Study the drawing (mm; zero at the part's minimum x, y, z) and answer. A direction names the side the tool comes from. Coordinates: 2 decimals unless noted, no trailing zeros. Loops run counter-clockwise (first coordinate to the right, second up) from the corner with the lowest first, then second, coordinate; pieces in that order, holes last. Notation, with made-up numbers: (70.25, -14) - (106.25, -14) arc R24 cw to (106.25, 24) - close; hole circle Ø3 at (55, -39.5). An arc over 180 degrees is marked (long way). Use one line per item in the form item = value.
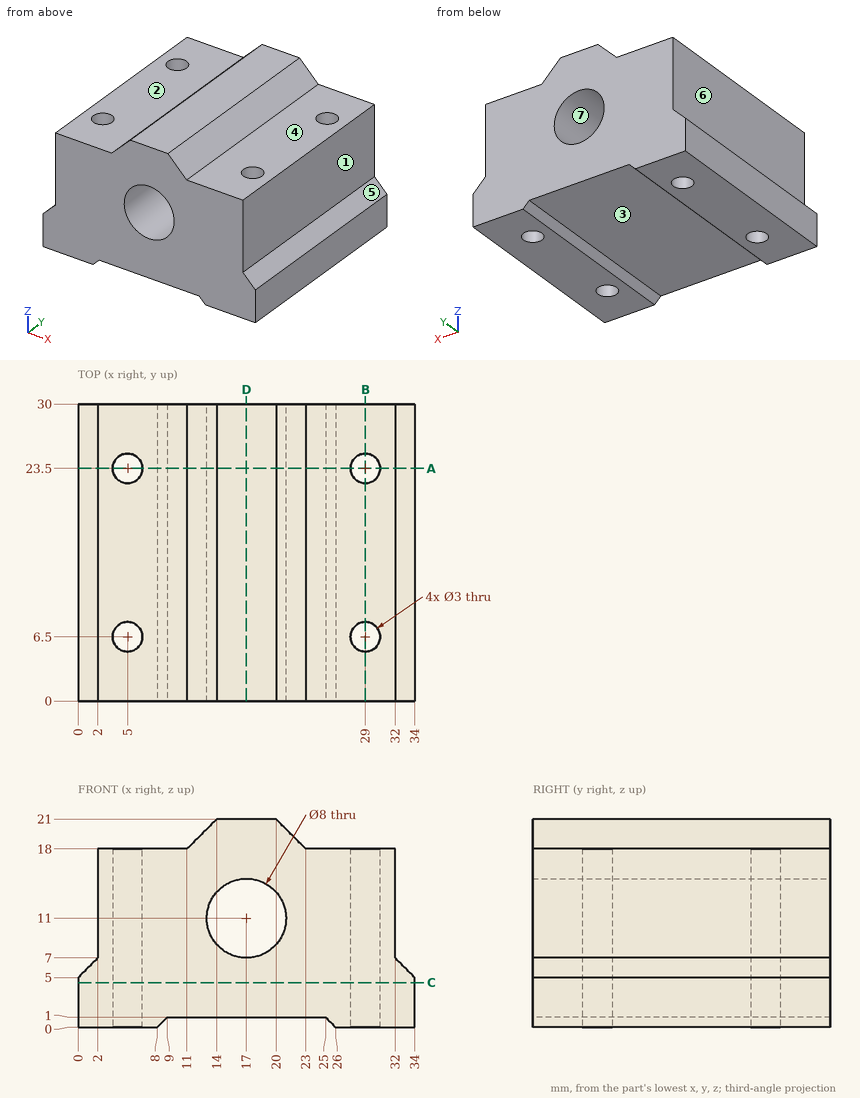
Item 1: Which of the six approach directions +Z, -Z, +X, -X, +Y, -Y give full straight-line access (tool end or side, diameter ignored) to the marked faces 1, 2 and 3?
Results below:
face_1 = +Z, +X, +Y, -Y
face_2 = +Z, -X, +Y, -Y
face_3 = -Z, +Y, -Y
Item 2: Find the intervals of material crossed by L1, parallel to Y at x = 5, z = 12.75; L2, parallel to X at y = 6.5, z = 3.75; L3, parallel to X at y = 9, z = 11, in increasing order.
Results below:
L1 = 0 to 5, 8 to 22, 25 to 30
L2 = 0 to 3.5, 6.5 to 27.5, 30.5 to 34
L3 = 2 to 13, 21 to 32
Item 3: Each of these flat-tipped pins is pushed along its axis until it touches: P1, Ø10, axis at x = 29, y = 16.5, coming from the +Z side; P2, Ø1.5, axis at x = 14, y = 20, coming from the -Z side; P3, Ø9, axis at y = 8, z = 14, coming from the -X side. Where does it stop, or does it pass through?
Results below:
P1 = 18
P2 = 1
P3 = 2
Item 4: The part is cut by section D-D on x = 17. Give the vertices of the cut face in (y, z), plus the area to 3 significant figures.
Results below:
outline = (0, 1) - (30, 1) - (30, 7) - (0, 7) - close; (0, 15) - (30, 15) - (30, 21) - (0, 21) - close
area = 360 mm²
Item 5: The part is cut by section C-C on z = 4.5. Give the vertices of the cut face in (x, y).
Results below:
outline = (0, 0) - (34, 0) - (34, 30) - (0, 30) - close; hole circle Ø3 at (5, 6.5); hole circle Ø3 at (5, 23.5); hole circle Ø3 at (29, 6.5); hole circle Ø3 at (29, 23.5)
Item 6: The part is cut by section B-B on x = 29. Give the vertices of the cut face in (y, z).
Results below:
outline = (0, 0) - (5, 0) - (5, 18) - (0, 18) - close; (8, 0) - (22, 0) - (22, 18) - (8, 18) - close; (25, 0) - (30, 0) - (30, 18) - (25, 18) - close
Item 7: The part is cut by section A-A on y = 23.5. Give the vertices of the cut face in (x, z).
Results below:
outline = (0, 0) - (3.5, 0) - (3.5, 18) - (2, 18) - (2, 7) - (0, 5) - close; (6.5, 0) - (8, 0) - (9, 1) - (25, 1) - (26, 0) - (27.5, 0) - (27.5, 18) - (23, 18) - (20, 21) - (14, 21) - (11, 18) - (6.5, 18) - close; (30.5, 0) - (34, 0) - (34, 5) - (32, 7) - (32, 18) - (30.5, 18) - close; hole circle Ø8 at (17, 11)
Item 8: For a pull along X with two mould halves and no side action, classify the marked faces 4, 5, 6 and 7 as +X half, -X half, draft (parallel to the pull), parting line (faces both ways), or undercut.
Results below:
face_4 = draft
face_5 = +X half
face_6 = -X half
face_7 = undercut
